```python
from build123d import *

# Parameters (mm, degrees)
F0_W     = 104.775
F0_H     = 63.5
F1_DEPTH = 47.625
F2_R     = 12.7
F3_DEPTH = 47.625
F5_DEPTH = 47.625


with BuildPart() as f1:
    # F0 (on Front) → F1 (new body)
    with BuildSketch(Plane.XZ):
        with Locations((17.757324, 1.931498)):
            Rectangle(F0_W, F0_H)
        with BuildLine():
            Line((-34.630176, -29.818502), (-34.630176, 33.681498))
            ThreePointArc((-34.630176, 33.681498), (-66.380176, 1.931498), (-34.630176, -29.818502))
        make_face()
    extrude(amount=F1_DEPTH)

    # F2 (on face) → F3 (cut)
    with BuildSketch(Plane.XZ.offset(47.625)):
        with Locations((-34.630176, 1.931498)):
            Circle(F2_R)
    extrude(amount=-F3_DEPTH, mode=Mode.SUBTRACT)

    # F4 (on face) → F5 (cut)
    with BuildSketch(Plane.XZ.offset(47.625)):
        with BuildLine():
            Line((70.144824, 33.681498), (38.394824, 33.681498))
            ThreePointArc((38.394824, 33.681498), (47.694183, 11.230857), (70.144824, 1.931498))
            Line((70.144824, 1.931498), (70.144824, 33.681498))
        make_face()
    extrude(amount=-F5_DEPTH, mode=Mode.SUBTRACT)


solid = f1.part
```
Source: CAD feature listing. Evaluate the final solid. Frame: model axes, mm. Give positions to 0.01 mm unless a question says otherwise; leave off trailing zeros. Write each loop counter-clockwise with the first axis right and the second up, starting at its lowest first coordinate (ties: lowest second). Pieces come first, ordered by that corner, then holes. Notation, with made-up numbers: (37.5, 57.25) - (75.5, 57.25) arc R30 cw to (75.5, 95.25) - close; hole circle Ø8 at (50, -16.5). An arc over 180 degrees is marked (long way). One line per item, written item: value. Start each with the question number.
Q1. Section query D-D, the plane z = 21. Return the cut outline in (x, y) (3 decimals), then the cut area to 3 significant figures.
Q2. First-contact query: pin 1 Ø23 at (x, z) = (-34.63, 1.93) entering from +Y; pin 2 Ø12 at (y, z) = (-30, 0) entering from -X. Flat tips, straight axial feed; report the tip coordinate or a pass-through.
Q3. Draft query along Z for faces 1 (the face through (17, -23, -29.819)), 2 (the face through (1, -47.625, 2)), 3 (the face through (-22.517, -24.146, 5.746)), 4 (the face through (-66.372, -23.479, 2.63)). Return one class per face: +Z half, -Z half, draft (parallel to the pull), parting line (faces both ways), or undercut.
Q4. Section query A-A, the plane x = -41.5. Return the cut outline in (y, z) (3 decimals), then the cut area to 3 significant figures.
Q5. Section query C-C, the plane y = -13.5. Return the cut outline in (x, z).
Q6. Section query B-B, the plane z = -9. Return the cut outline in (x, y) (3 decimals), then the cut area to 3 significant figures.
Q7. Material intervals for probe 1 along X at (y, z) = (-5.5, 12.5); probe 2 along X at (y, z) = (-41, -6.5); probe 3 along Z at (x, y) = (-57, -21.5), sorted ascending. Write a range as from..to.
Answer:
1. outline: (-60.016, -47.625) - (41.037, -47.625) - (41.037, 0) - (-60.016, 0) - close
1. area: 4,810 mm2
2. pin 1: passes through
2. pin 2: stops at x = -66.38
3. face 1: -Z half
3. face 2: draft
3. face 3: undercut
3. face 4: parting line
4. outline: (-47.625, -29.066) - (0, -29.066) - (0, -8.75) - (-47.625, -8.75) - close; (-47.625, 12.613) - (0, 12.613) - (0, 32.929) - (-47.625, 32.929) - close
4. area: 1,940 mm2
5. outline: (-34.63, -29.82) - (70.14, -29.82) - (70.14, 1.93) arc R31.75 cw to (38.39, 33.68) - (-34.63, 33.68) arc R31.75 ccw to start; hole circle Ø25.4 at (-34.63, 1.93)
6. outline: (-64.439, -47.625) - (-41.095, -47.625) - (-41.095, 0) - (-64.439, 0) - close; (-28.165, -47.625) - (70.145, -47.625) - (70.145, 0) - (-28.165, 0) - close
6. area: 5,790 mm2
7. probe 1: x = -64.57..-41.67, -27.59..46.49
7. probe 2: x = -65.24..-44.13, -25.13..70.14
7. probe 3: z = -20.6..24.46
